Work out the finished part from the listing and answer in its coordinate system (mm). Face numbers are marked on the shaded views. Coordinates: 2 decimals unless noted, no trailing zeros. Order: outer loops, then holes, each group sorted by start corner. A loop starts at its lowest first (then second) coordinate and runs counter-clockwise, first axis right, second up. Notation, with made-up numbers: (58.25, 31) -> (108.25, 31) arc R21 cw to (108.25, 42) -> close; hole circle Ø7 at (-24.5, -0.75). An arc over 180 degrees is marked (long way). Write item = value, one per line. Start each with the question number.
Q1. Straight lines are drawn through the part: L1, parallel to Y at x = 0, z = 12; L2, parallel to X at y = 0.5, z = 10; L3, parallel to Y at x = -19, z = 6.25. For each, find the intervals that lie inside material, in ascending order. Write a range as from..to.
Q2. The part is cut by section C-C, the plane z = 23. Count the separate pieces of the cut face and the enclosed holes in it, plus the area to 3 significant figures.
Q3. For a pull along Y with two mould halves and no side action, classify the marked faces 1, 2 and 3 as +Y half, -Y half, draft (parallel to the pull), parting line (faces both ways), or undercut.
Q4. The part is cut by section A-A, the plane x = 0. Determine the outline of the cut face in (y, z), plus the area to 3 significant figures.
Q5. Flat-ended cylindrical pins translate along their axes: pin 1 (5 mm diameter, centred on y = -13.5, z = 19, fed in from +X); pin 2 (8 mm diameter, centred on x = 3, z = 16, fed in from +Y); pin 3 (2 mm diameter, centred on y = -12.5, z = 22.5, fed in from -X). Find the tip coordinate at first contact, or state that the pin passes through.
Q6. The part is cut by section D-D, the plane x = 19.05. Determine the outline of the cut face in (y, z).
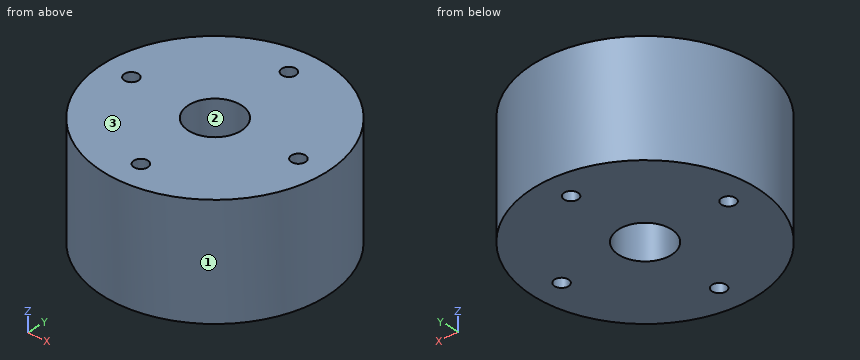
```python
from build123d import *

# Parameters (mm, degrees)
F0_R     = 25.4
F0_R_2   = 1.5875
F0_R_3   = 6
F1_DEPTH = 19.05
F2_DEPTH = 25.4


with BuildPart() as f1:
    # F0 (on Top) → F1 (new body)
    with BuildSketch(Plane.XY):
        Circle(F0_R)
        with Locations((0, -19.05)):
            Circle(F0_R_2, mode=Mode.SUBTRACT)
        with Locations((-19.05, 0)):
            Circle(F0_R_2, mode=Mode.SUBTRACT)
        Circle(F0_R_3, mode=Mode.SUBTRACT)
        with Locations((19.05, 0)):
            Circle(F0_R_2, mode=Mode.SUBTRACT)
        with Locations((0, 19.05)):
            Circle(F0_R_2, mode=Mode.SUBTRACT)
    extrude(amount=F1_DEPTH)

    # F0 (on Top) → F2 (join)
    with BuildSketch(Plane.XY):
        Circle(F0_R)
        with Locations((0, -19.05)):
            Circle(F0_R_2, mode=Mode.SUBTRACT)
        with Locations((-19.05, 0)):
            Circle(F0_R_2, mode=Mode.SUBTRACT)
        Circle(F0_R_3, mode=Mode.SUBTRACT)
        with Locations((19.05, 0)):
            Circle(F0_R_2, mode=Mode.SUBTRACT)
        with Locations((0, 19.05)):
            Circle(F0_R_2, mode=Mode.SUBTRACT)
    extrude(amount=F2_DEPTH)


solid = f1.part
```
Model answer:
q1.L1 = -25.4..-20.64, -17.46..-6, 6..17.46, 20.64..25.4
q1.L2 = -25.4..-20.56, -17.54..-5.98, 5.98..17.54, 20.56..25.4
q1.L3 = -16.86..-1.59, 1.59..16.86
q2.separate_pieces = 1
q2.enclosed_holes = 5
q2.area = 1,880 mm2
q3.face_1 = parting line
q3.face_2 = undercut
q3.face_3 = draft
q4.outline = (-25.4, 0) -> (-20.64, 0) -> (-20.64, 25.4) -> (-25.4, 25.4) -> close; (-17.46, 0) -> (-6, 0) -> (-6, 25.4) -> (-17.46, 25.4) -> close; (6, 0) -> (17.46, 0) -> (17.46, 25.4) -> (6, 25.4) -> close; (20.64, 0) -> (25.4, 0) -> (25.4, 25.4) -> (20.64, 25.4) -> close
q4.area = 824 mm2
q5.pin_1 = 22.89
q5.pin_2 = 25.4
q5.pin_3 = -22.65
q6.outline = (-16.8, 0) -> (-1.59, 0) -> (-1.59, 25.4) -> (-16.8, 25.4) -> close; (1.59, 0) -> (16.8, 0) -> (16.8, 25.4) -> (1.59, 25.4) -> close
